Part model, mm, in its own coordinate system. A direction names the side the tool comes from. Coordinates: 2 decimals unless noted, no trailing zeros. Loops run counter-clockwise (first coordinate to the right, second up) from the corner with the lowest first, then second, coordinate; pieces in that order, holes last.
```python
from build123d import *

# Parameters (mm, degrees)
SKETCH_1_W          = 12.8
SKETCH_1_H          = 44.8
EXTRUDE_1_DEPTH     = 12.7
SKETCH_2_R          = 2.2
CUT_EXTRUDE_1_DEPTH = 36.575886954
SKETCH_3_R          = 2.2
CUT_EXTRUDE_2_DEPTH = 33.16376457
SKETCH_4_R          = 2.2
CUT_EXTRUDE_3_DEPTH = 51.629102117
CUT_EXTRUDE_4_DEPTH = 3.5
CUT_EXTRUDE_5_DEPTH = 3.5
CUT_EXTRUDE_6_DEPTH = 3.5
CUT_EXTRUDE_7_DEPTH = 3.5


with BuildPart() as part:
    # 草圖1 → 填料-伸長1 (new body)
    with BuildSketch(Plane.XY):
        with Locations((13.474002647, -4.234146341)):
            Rectangle(SKETCH_1_W, SKETCH_1_H)
    extrude(amount=EXTRUDE_1_DEPTH)

    # 草圖2 → 除料-伸長1 (cut, through all)
    with BuildSketch(Plane.XY.offset(12.7)):
        with Locations((13.474002647, -4.234146341)):
            Circle(SKETCH_2_R)
    extrude(amount=-CUT_EXTRUDE_1_DEPTH, mode=Mode.SUBTRACT)

    # 草圖3 → 除料-伸長2 (cut, through all)
    with BuildSketch(Plane.ZY.offset(-7.074002647)):
        with Locations(Location((6.35, 3.765853659, 0), (0, 0, 270))):
            Circle(SKETCH_3_R)
        with Locations(Location((6.35, -12.234146341, 0), (0, 0, 270))):
            Circle(SKETCH_3_R)
    extrude(amount=-CUT_EXTRUDE_2_DEPTH, mode=Mode.SUBTRACT)

    # 草圖4 → 除料-伸長3 (cut, through all)
    with BuildSketch(Plane(origin=(0, 18.165853659, 0), x_dir=(1, 0, 0), z_dir=(0, 1, 0))):
        with Locations(Location((13.474002647, -6.35, 0), (0, 0, 180))):
            Circle(SKETCH_4_R)
    extrude(amount=-CUT_EXTRUDE_3_DEPTH, mode=Mode.SUBTRACT)

    # 草圖5 → 除料-伸長4 (cut)
    with BuildSketch(Plane.XY.offset(12.7)):
        Polygon((9.221190711, -5.048757069), (12.053070264, -8.324494879), (16.3058822, -7.509884151), (17.726814583, -3.419535613), (14.89493503, -0.143797803), (10.642123094, -0.958408532), align=None)
    extrude(amount=-CUT_EXTRUDE_4_DEPTH, mode=Mode.SUBTRACT)

    # 草圖6 → 除料-伸長5 (cut)
    with BuildSketch(Plane.ZY.offset(-7.074002647)):
        Polygon((9.740257522, -14.92787126), (10.377962971, -10.644959661), (6.987705449, -7.951234743), (2.959742478, -9.540421423), (2.322037029, -13.823333022), (5.712294551, -16.51705794), align=None)
        Polygon((9.740257522, 1.07212874), (10.377962971, 5.355040339), (6.987705449, 8.048765257), (2.959742478, 6.459578577), (2.322037029, 2.176666978), (5.712294551, -0.51705794), align=None)
    extrude(amount=-CUT_EXTRUDE_5_DEPTH, mode=Mode.SUBTRACT)

    # 草圖7 → 除料-伸長6 (cut)
    with BuildSketch(Plane.XZ.offset(26.634146341)):
        Polygon((17.407945653, 4.540554664), (17.007999778, 8.852171913), (13.074056771, 10.661617248), (9.540059641, 8.159445336), (9.940005516, 3.847828087), (13.873948523, 2.038382752), align=None)
    extrude(amount=-CUT_EXTRUDE_6_DEPTH, mode=Mode.SUBTRACT)

    # 草圖8 → 除料-伸長7 (cut)
    with BuildSketch(Plane(origin=(0, 18.165853659, 0), x_dir=(1, 0, 0), z_dir=(0, 1, 0))):
        Polygon((14.348050125, -10.590995285), (17.58383604, -7.713550322), (16.709788562, -3.472555037), (12.599955169, -2.109004715), (9.364169254, -4.986449678), (10.238216732, -9.227444963), align=None)
    extrude(amount=-CUT_EXTRUDE_7_DEPTH, mode=Mode.SUBTRACT)


solid = part.part
```
Q1. Tool access for faces 1 (the flat face through (11.332, -24.909, 9.428)), 2 (the flat face through (12.798, -0.545, 10.974)), 3 (the flat face through (8.8, 6.68, 8.71)): list every direction of +Z, -Z, +X, -X, +Y, -Y with a clear straight run to the whole face (end or side of a thin tool).
Q2. Saw through at B-B (z = 1.5). List the corners of the cut face in (x, y).
Q3. Probe line 1 (Y direction, x = 15.75, z = 6.5); line 2 (Y direction, x = 19.5, z = 7.75); line 3 (X direction, y = -11, z = 9). List the from-to ranges inside material, lowest first.
Q4. Saw through at A-A (y = -19). List the corners of the cut face in (x, z), plus the area to 3 significant figures.
Q5. Saw through at C-C (y = -2.5). List the corners of the cut face in (x, z), plus the area to 3 significant figures.
Q6. Mould opens along X. For faces 4 (the flat face through (8.8, -12.816, 10.055)), 5 (the flat face through (7.074, -5, 6)), 6 (the flat face through (15.069, -24.909, 9.744)) say: released by +X, released by -X, zero draft, split by the parting line, or undercut.
Q7. Drop flat-ended pins along their axis: P1, Ø5, axis at x = 13.47, y = -4.23, coming from the +Z side; P2, Ø7, axis at y = 3.77, z = 6.35, coming from the -X side; P3, Ø7, axis at x = 13.47, z = 6.35, coming from the +Y side. Give the stop position or say it passes through.
Checked values:
1. face 1: -Y
1. face 2: +Z
1. face 3: -X
2. outline: (7.07, -26.63) - (19.87, -26.63) - (19.87, 18.17) - (7.07, 18.17) - close; hole circle Ø4.4 at (13.47, -4.23)
3. line 1: y = -23.13 to -14.43, -10.04 to 1.57, 5.96 to 14.67
3. line 2: y = -26.63 to -13.93, -10.54 to 2.07, 5.46 to 18.17
3. line 3: x = 10.57 to 19.87
4. outline: (7.07, 0) - (19.87, 0) - (19.87, 12.7) - (7.07, 12.7) - close; hole circle Ø4.4 at (13.47, 6.35)
4. area: 147 mm2
5. outline: (7.07, 0) - (12.12, 0) - (12.12, 4.62) arc R2.2 cw to (12.12, 8.08) - (12.12, 9.2) - (10.11, 9.2) - (10.11, 12.7) - (7.07, 12.7) - close; (14.83, 0) - (19.87, 0) - (19.87, 12.7) - (16.93, 12.7) - (16.93, 9.2) - (14.83, 9.2) - (14.83, 8.08) arc R2.2 cw to (14.83, 4.62) - close
5. area: 110 mm2
6. face 4: zero draft
6. face 5: released by -X
6. face 6: undercut
7. P1: stops at z = 9.2
7. P2: stops at x = 10.57
7. P3: stops at y = 14.67
